Geometry: final body of the model. Coordinates: model frame, mm. A direction names the side the tool comes from. Round coordinates to 2 decimals unless told otherwise and drop trailing zeros. Return JSON: item names as keys, results as strings. Group by question number.
1. Set-up query: faces 3 (the face through (8.962, 108.874, 0.32)), 4 (the face through (17.663, 188.654, 4.196)), 5 (the face through (-27, 99, -8.87)), 6 (the face through (-6.58, 94, -2.78)). Return all of +Z, -Z, +X, -X, +Y, -Y with unobstructed straight access to the full face (end or side cutting, diameter ignored); none if empty.
2. Material intervals for probe 1 along Y at (x, z) = (21.16, 7.75) (3 decimals); probe 2 along Y at (x, z) = (21.16, 3.85); probe 3 along Y at (x, z) = (-1, 4.5), sorted ascending.
3. Draft query along Y for faces 1 (the face through (8.39, 98.865, -0.297)), 2 (the face through (-27, 6, 5.87)). Return one class per face: +Y half, -Y half, draft (parallel to the pull), parting line (faces both ways), or undercut.
4. First-contact query: pin 1 Ø3.5 at (x, y) = (23, 189.5) entering from -Z; pin 2 Ø1.5 at (x, z) = (-56, -7) entering from +Y; pin 3 Ø0.6 at (x, z) = (-57, -5) entering from -Y. Flat tips, straight axial feed; report the tip coordinate or a pass-through.
from build123d import *

# Parameters (mm, degrees)
CROQUIS1_W                 = 78.58
CROQUIS1_H                 = 17.74
SALIENTE_EXTRUIR1_DEPTH    = 195
CORTAR_EXTRUIR1_DEPTH      = 200.116501074
CORTAR_EXTRUIR1_DEPTH_BACK = 200.116501074
CHAFL_N1_SIZE2             = 3.821967962
CHAFL_N1_SIZE              = 3
CROQUIS4_W                 = 3
CROQUIS4_H                 = 195
SALIENTE_EXTRUIR2_DEPTH    = 3
CROQUIS5_W                 = 25.18
CROQUIS5_H                 = 143
SALIENTE_EXTRUIR3_DEPTH    = 3
REDONDEO1_R                = 2
CORTAR_EXTRUIR2_DEPTH      = 208.103617786
CORTAR_EXTRUIR2_DEPTH_BACK = 208.103617786
CROQUIS6_R                 = 1.625
CORTAR_EXTRUIR3_START      = -3
CROQUIS7_R                 = 3.5
CORTAR_EXTRUIR3_DEPTH      = 205.103617786
CROQUIS8_R                 = 16.25
CROQUIS8_R_2               = 8.75
CORTAR_EXTRUIR4_DEPTH      = 3
CROQUIS9_R                 = 17.25
SALIENTE_EXTRUIR4_DEPTH    = 2
CHAFL_N2_SIZE              = 2
CORTAR_EXTRUIR6_DEPTH      = 208.103617786
CORTAR_EXTRUIR6_DEPTH_BACK = 208.103617786
CROQUIS10_W                = 3.5
CROQUIS10_H                = 9
CORTAR_EXTRUIR7_DEPTH      = 1
CORTAR_EXTRUIR8_START      = -13
CORTAR_EXTRUIR8_DEPTH      = 169


with BuildPart() as part:
    # Croquis1 → Saliente-Extruir1 (new body)
    with BuildSketch(Plane(origin=(0, 0, 0), x_dir=(1, 0, 0), z_dir=(0, 1, 0))):
        Rectangle(CROQUIS1_W, CROQUIS1_H)
    extrude(amount=SALIENTE_EXTRUIR1_DEPTH)

    # Croquis2 → Cortar-Extruir1 (cut, two sides: drawn at the far end of the back side and taken through both)
    with BuildSketch(Plane.XZ.offset(-CORTAR_EXTRUIR1_DEPTH_BACK)):
        Polygon((39.29, 5.87), (-19.532543769, -5.87), (-19.532543769, -8.87), (39.29, -8.87), align=None)
    extrude(amount=CORTAR_EXTRUIR1_DEPTH + CORTAR_EXTRUIR1_DEPTH_BACK, mode=Mode.SUBTRACT)

    # Chaflán1
    chafl_n1_edges = [part.edges().sort_by_distance(p)[0] for p in [
        (39.29, 97.5, 5.87),
    ]]
    chafl_n1_side = [part.faces().sort_by_distance(p)[0] for p in [
        (39.29, 97.5, 5.93),
    ]]
    chamfer(chafl_n1_edges, length=CHAFL_N1_SIZE - 0.0001, length2=CHAFL_N1_SIZE2 - 0.0001, reference=chafl_n1_side[0])  # a hair under: the kernel refuses the full size

    # Croquis4 → Saliente-Extruir2 (add)
    with BuildSketch(Plane(origin=(0, 0, -8.87), x_dir=(-1, 0, 0), z_dir=(0, 0, -1))):
        with Locations((40.79, 97.5)):
            Rectangle(CROQUIS4_W, CROQUIS4_H)
    extrude(amount=-SALIENTE_EXTRUIR2_DEPTH)

    # Croquis5 → Saliente-Extruir3 (add)
    with BuildSketch(Plane(origin=(0, 0, -8.87), x_dir=(-1, 0, 0), z_dir=(0, 0, -1))):
        with Locations((54.88, 97.5)):
            Rectangle(CROQUIS5_W, CROQUIS5_H)
    extrude(amount=-SALIENTE_EXTRUIR3_DEPTH)

    # Redondeo1
    redondeo1_edges = [part.edges().sort_by_distance(p)[0] for p in [
        (-67.47, 97.5, -8.87),
    ]]
    fillet(redondeo1_edges, radius=REDONDEO1_R)

    # Croquis6 → Cortar-Extruir2 (cut, two sides: drawn at the far end of the back side and taken through both)
    with BuildSketch(Plane.XY.offset(8.87).offset(-CORTAR_EXTRUIR2_DEPTH_BACK)):
        with Locations((-28.84, 188.5)):
            Circle(CROQUIS6_R)
        with Locations((21.16, 188.5)):
            Circle(CROQUIS6_R)
        with Locations((21.16, 6.5)):
            Circle(CROQUIS6_R)
        with Locations(Location((-28.84, 6.5, 0), (0, 0, 180))):
            Circle(CROQUIS6_R)
    extrude(amount=CORTAR_EXTRUIR2_DEPTH + CORTAR_EXTRUIR2_DEPTH_BACK, mode=Mode.SUBTRACT)

    # Croquis7 → Cortar-Extruir3 (cut, through all)
    with BuildSketch(Plane.XY.offset(8.87).offset(CORTAR_EXTRUIR3_START)):
        with Locations((-28.84, 188.5)):
            Circle(CROQUIS7_R)
        with Locations((21.16, 188.5)):
            Circle(CROQUIS7_R)
        with Locations((-28.84, 6.5)):
            Circle(CROQUIS7_R)
        with Locations((21.16, 6.5)):
            Circle(CROQUIS7_R)
    extrude(amount=-CORTAR_EXTRUIR3_DEPTH, mode=Mode.SUBTRACT)

    # Croquis8 → Cortar-Extruir4 (cut)
    with BuildSketch(Plane(origin=(0, 0, -8.87), x_dir=(-1, 0, 0), z_dir=(0, 0, -1))):
        with Locations((44.469949206, 97.5)):
            Circle(CROQUIS8_R)
        with Locations((44.469949206, 97.5)):
            Circle(CROQUIS8_R_2, mode=Mode.SUBTRACT)
    extrude(amount=-CORTAR_EXTRUIR4_DEPTH, mode=Mode.SUBTRACT)

    # Croquis9 → Saliente-Extruir4 (add)
    with BuildSketch(Plane.XY.offset(-5.87)):
        with Locations((-44.469949206, 97.5)):
            Circle(CROQUIS9_R)
    extrude(amount=SALIENTE_EXTRUIR4_DEPTH)

    # Chaflán2
    chafl_n2_edges = [part.edges().sort_by_distance(p)[0] for p in [
        (-61.719949206, 97.5, -5.87),
    ]]
    chamfer(chafl_n2_edges, length=CHAFL_N2_SIZE - 0.0001)  # a hair under: the kernel refuses the full size

    # Croquis10 → Cortar-Extruir6 (cut, two sides: drawn at the far end of the back side and taken through both)
    with BuildSketch(Plane(origin=(0, 0, -8.87), x_dir=(-1, 0, 0), z_dir=(0, 0, -1)).offset(-CORTAR_EXTRUIR6_DEPTH_BACK)):
        with Locations((57.22, 99)):
            Rectangle(CROQUIS10_W, CROQUIS10_H)
    extrude(amount=CORTAR_EXTRUIR6_DEPTH + CORTAR_EXTRUIR6_DEPTH_BACK, mode=Mode.SUBTRACT)

    # Croquis11 → Cortar-Extruir7 (cut)
    with BuildSketch(Plane(origin=(0.378430223, 0, -1.896101224), x_dir=(-0.9806591733939511, 0, -0.1957232373487947), z_dir=(0.19572323734879468, 0, -0.980659173393951))):
        Polygon((-28.864838216, 97.5), (-15.458781877, 92.947300595), (-7.58538371, 97.5), (-15.458781877, 102.052699405), align=None)
        Polygon((-10.689272405, 88.750905342), (-6.961025568, 83.426417054), (-14.813228871, 81.895762524), align=None)
        Polygon((-8.5598171, 92.683515176), (-1.676899864, 82.853690645), (9.381652734, 90.596972535), (4.548100867, 97.5), (9.381652734, 104.403027465), (-1.676899864, 112.146309355), (-8.5598171, 102.316484824), (-2.496901935, 106.616608043), (2.418010331, 103.175149425), (-1.555772077, 97.5), (2.418010331, 91.824850575), (-2.496901935, 88.383391957), align=None)
        Polygon((7.048100867, 97.5), (9.548100867, 95), (14.008259291, 97.5), (9.548100867, 100), align=None)
        Polygon((-14.813228871, 113.104237476), (-10.689272405, 106.249094658), (-6.961025568, 111.573582946), align=None)
    extrude(amount=-CORTAR_EXTRUIR7_DEPTH, mode=Mode.SUBTRACT)

    # Croquis12 → Cortar-Extruir8 (cut)
    with BuildSketch(Plane.XZ.offset(CORTAR_EXTRUIR8_START)):
        Polygon((-20.119713481, -2.92802248), (-24.839433576, -3.87), (-39.29, -3.87), (-39.29, 8.87), (35.047359313, 8.87), (34.063379787, 7.886020474), align=None)
    extrude(amount=-CORTAR_EXTRUIR8_DEPTH, mode=Mode.SUBTRACT)


solid = part.part
Taken from the geometry:
{
 "1": {"face 3": "none", "face 4": "-Z", "face 5": "-Z, +X, -X, +Y, -Y", "face 6": "+X"},
 "2": {"probe 1": "0 to 4.875, 8.125 to 13, 182 to 186.875, 190.125 to 195", "probe 2": "0 to 3, 10 to 185, 192 to 195", "probe 3": "0 to 13, 182 to 195"},
 "3": {"face 1": "draft", "face 2": "undercut"},
 "4": {"pin 1": "z = 2.69", "pin 2": "y = 169", "pin 3": "y = 83.56"}
}
